Part print with two shaded views. Sizes in mm from the minimum x, y, z corner. A direction names the side the tool comes from. Give positions to 0.01 mm unless a question says otherwise; leave off trailing zeros. Write each loop counter-clockwise with the first axis right and the second up, starting at its lowest first coordinate (ties: lowest second). Pieces come first, ordered by that corner, then holes. Notation, with made-up numbers: M 68,-20.5 L 82,-20.5 A12 ccw 82,-6.5 Z; hole C 49.5,46 d5. An arc over 180 degrees is marked long. Return JSON: item names as keys, results as strings. Group by question number.
Q1. Band-saw the part on C-C, the plane x = 16.5. Give the cut face in (y, z), then the cut area to 3 significant figures.
Q2. Band-saw the part on A-A, the plane z = 4. Give the cut face in (x, y).
Q3. Flat gauge pins, fed straight in: pin 1 Ø5 at (x, y) = (53.5, 2.5) entering from +Z; pin 2 Ø5 at (x, y) = (67.5, 18.5) entering from -Z; pin 3 Ø1.5 at (y, z) = (2.5, 35.5) entering from -X. Where does each tip first touch, or does it go through?
Q4. Pull direction Z, two halves, no side cores. Call the marked faces 4, 5 and 6: +Z half, -Z half, draft (parallel to the pull), parting line (faces both ways), or undercut.
Q5. Band-saw the part on B-B, the plane y = 7.25. Give the cut face in (x, z).
Q6. Band-saw the part on D-D, the plane z = 32. Give the cut face in (x, y), then the cut area to 3 significant figures.
Q7. Wall check: probe 1 along X at (y, z) = (3.25, 32); probe 2 along X at (y, z) = (6, 32); probe 3 along X at (y, z) = (17.75, 26). Give the ranges that are in metal, low to high.
Q8. Tool access for the marked faces 1, 2 and 3: list every direction of +Z, -Z, +X, -X, +Y, -Y with a clear straight run to the whole face (end or side of a thin tool).
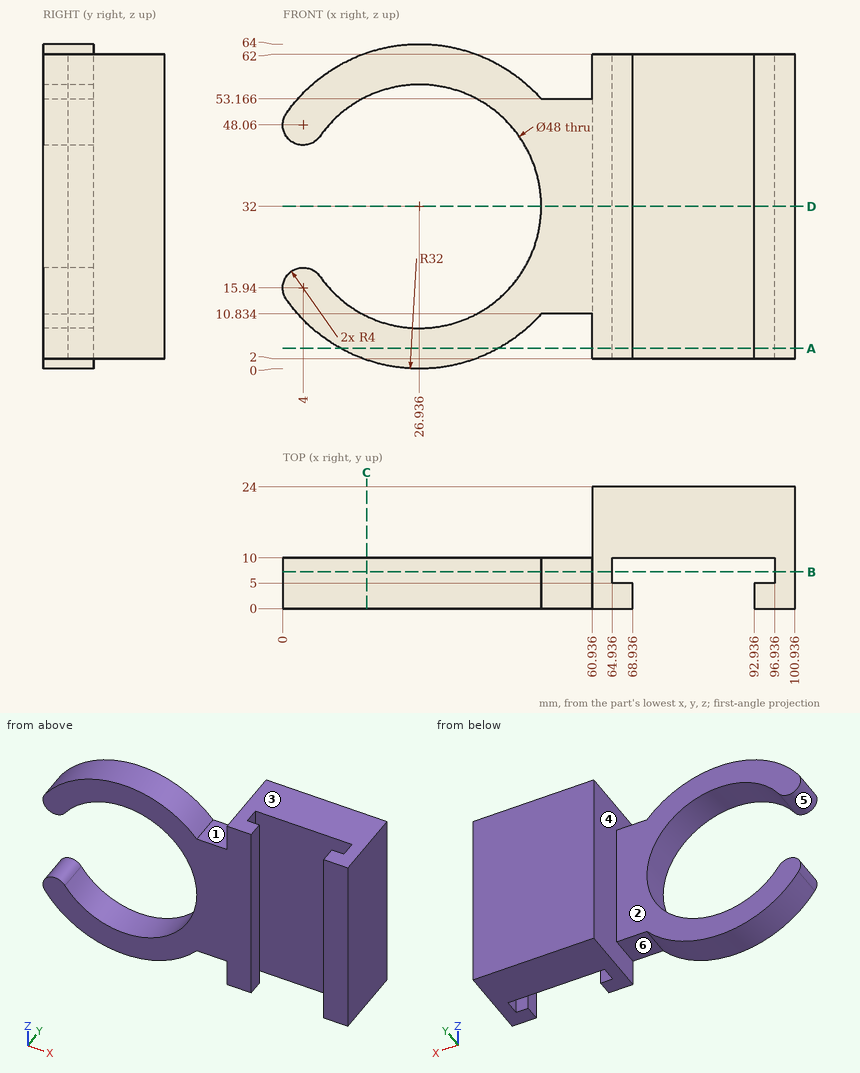
From the geometry:
{
 "1": {"outline": "M 0,1.75 L 10,1.75 L 10,10.39 L 0,10.39 Z; M 0,53.61 L 10,53.61 L 10,62.25 L 0,62.25 Z", "area": "173 mm^2"},
 "2": {"outline": "M 11.44,0 L 42.43,0 L 42.43,10 L 11.44,10 Z; M 60.94,0 L 68.94,0 L 68.94,5 L 64.94,5 L 64.94,10 L 96.94,10 L 96.94,5 L 92.94,5 L 92.94,0 L 100.94,0 L 100.94,24 L 60.94,24 Z"},
 "3": {"pin 1": "stops at z = 53.17", "pin 2": "stops at z = 2", "pin 3": "stops at x = 50.56"},
 "4": {"face 4": "draft", "face 5": "undercut", "face 6": "-Z half"},
 "5": {"outline": "M 0.72,13.65 A32 ccw 50.94,10.83 L 60.94,10.83 L 60.94,2 L 64.94,2 L 64.94,62 L 60.94,62 L 60.94,53.17 L 50.94,53.17 A32 ccw 0.72,50.35 A4 ccw 7.28,45.77 A24 cw long 7.28,18.23 A4 ccw Z; M 96.94,2 L 100.94,2 L 100.94,62 L 96.94,62 Z"},
 "6": {"outline": "M 50.94,0 L 68.94,0 L 68.94,5 L 64.94,5 L 64.94,10 L 96.94,10 L 96.94,5 L 92.94,5 L 92.94,0 L 100.94,0 L 100.94,24 L 60.94,24 L 60.94,10 L 50.94,10 Z", "area": "780 mm^2"},
 "7": {"probe 1": "x = 50.94 to 68.94, 92.94 to 100.94", "probe 2": "x = 50.94 to 64.94, 96.94 to 100.94", "probe 3": "x = 60.94 to 100.94"},
 "8": {"face 1": "+Z, +Y, -Y", "face 2": "+Z, -Z, -X, +Y", "face 3": "+Z, +X, +Y, -Y"}
}
